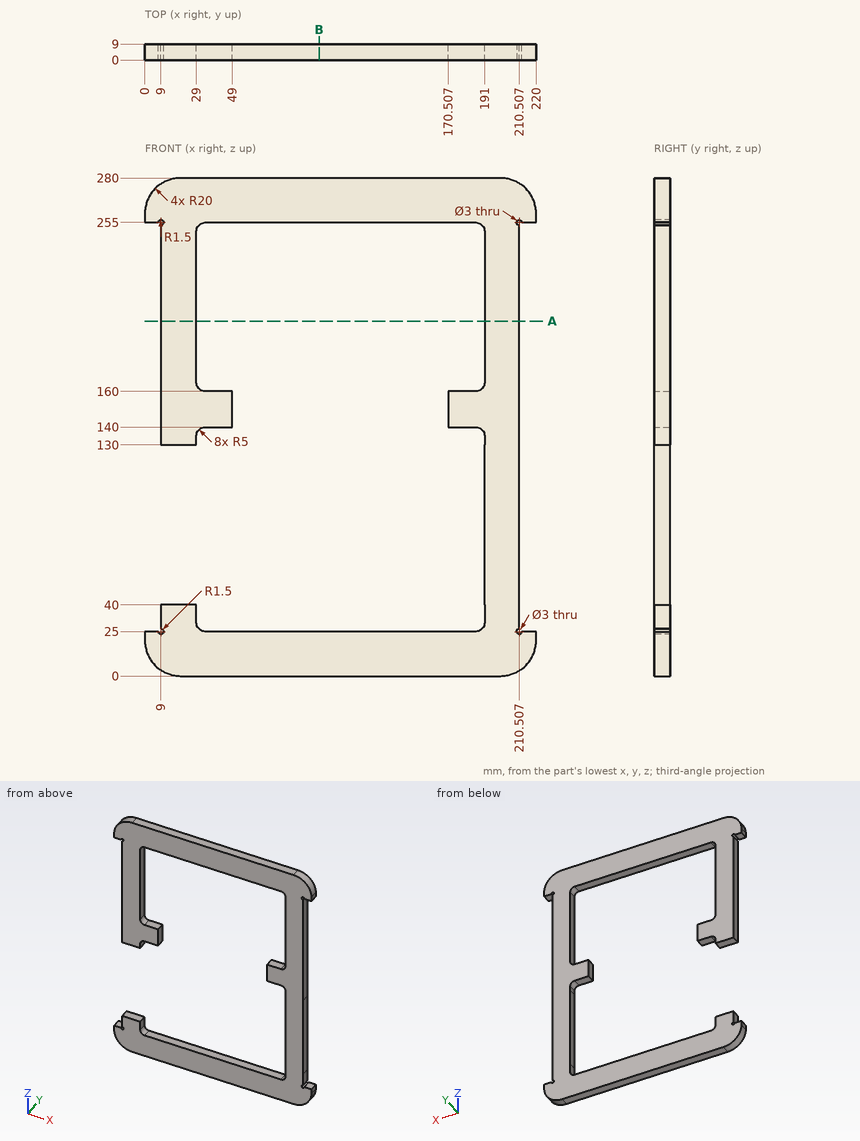
Check sheet for the drawn part. Datum: minimum x, y, z corner. Units: mm. Round coordinates to 2 decimals unless told otherwise and drop trailing zeros. Write each loop counter-clockwise with the first axis right and the second up, starting at its lowest first coordinate (ties: lowest second). Pieces come first, ordered by that corner, then holes. Notation, with made-up numbers: (-35.5, 21) -> (-29.5, 21) arc R28 cw to (-29.5, 46) -> close; hole circle Ø4 at (10.25, 11). An arc over 180 degrees is marked (long way). Write each question's results on one line, items separated by ' | '. Start each with the question number.
1. Material ranges on probe 1 along Z at (x, y) = (136, 7.25); probe 2 along X at (y, z) = (6.5, 154.5); probe 3 along X at (y, z) = (1, 250), recorded low to high. Write a range as from..to.
2. Depth check by flat-ended pin: P1, Ø5, axis at y = 3, z = 132, coming from the +X side; P2, Ø4.5, axis at y = 4, z = 150, coming from the -X side; P3, Ø4, axis at y = 5.5, z = 117, coming from the -X side; P4, Ø2, axis at x = 188.5, z = 109, coming from the -Y side. Enter the tip coordinate at first touch or a pass-through.
3. Cross-section at B-B (x = 98). Enter the section's corners in (y, z), then the cut area to 3 significant figures.
4. Cross-section at A-A (z = 199.5). Enter the section's corners in (x, y), then the cut area to 3 significant figures.
Solutions:
1) probe 1: z = 0..25, 255..280 | probe 2: x = 9..49, 170.51..210.51 | probe 3: x = 9..29, 191..210.51
2) P1: stops at x = 210.51 | P2: stops at x = 9 | P3: stops at x = 191 | P4: passes through
3) outline: (0, 0) -> (9, 0) -> (9, 25) -> (0, 25) -> close; (0, 255) -> (9, 255) -> (9, 280) -> (0, 280) -> close | area: 450 mm2
4) outline: (9, 0) -> (29, 0) -> (29, 9) -> (9, 9) -> close; (191, 0) -> (210.51, 0) -> (210.51, 9) -> (191, 9) -> close | area: 356 mm2
